Can you work these out from the model? Positions are in its coordinate system, mm. A direction names the side the tool comes from. Give positions to 0.01 mm unless a question says otherwise; leave off trailing zeros. Loops run counter-clockwise (first coordinate to the right, second up) from the corner with the lowest first, then second, coordinate; pieces in that order, holes last. Notation, with made-up numbers: M 72,79 L 123,79 A18 ccw 123,104 Z; hole C 75,7.5 d6. An arc over 180 degrees is marked long. One line per item, written item: value. Start each with the question number.
from build123d import *

# Parameters (mm, degrees)
F4_DEPTH = 2.794
F5_DEPTH = 25.4
F6_R     = 1.524
F7_DEPTH = 25.4
F9_DEPTH = 5.6388


with BuildPart() as f1:
    # F0 (on Front) → F1 (revolve)
    with BuildSketch(Plane.XZ):
        with BuildLine():
            Line((-42.70291, -13.129885), (-44.45, 0))
            Line((-44.45, 0), (-50.3936, 0))
            Line((-50.3936, 0), (-50.8, 0))
            Line((-50.8, 0), (-50.8, -0.4064))
            Line((-50.8, -0.4064), (-50.8, -5.238044))
            ThreePointArc((-50.8, -5.238044), (-50.680968, -5.525413), (-50.3936, -5.644444))
            Line((-50.3936, -5.644444), (-47.563638, -5.644444))
            ThreePointArc((-47.563638, -5.644444), (-47.006862, -5.875069), (-46.776238, -6.431844))
            Line((-46.776238, -6.431844), (-46.776238, -11.994444))
            Line((-46.776238, -11.994444), (-45.188738, -11.994444))
            Line((-45.188738, -11.994444), (-45.188738, -16.756944))
            Line((-45.188738, -16.756944), (-46.29761, -16.756944))
            ThreePointArc((-46.29761, -16.756944), (-46.558236, -16.898475), (-46.581447, -17.194142))
            Line((-46.581447, -17.194142), (-45.188738, -20.32))
            Line((-45.188738, -20.32), (-42.70291, -20.32))
            Line((-42.70291, -20.32), (-42.70291, -15.669885))
            Line((-42.70291, -15.669885), (0, -15.669885))
            Line((0, -15.669885), (0, -13.129885))
            Line((0, -13.129885), (-42.70291, -13.129885))
        make_face()
    revolve(axis=Axis((0, 0, -10.16), (0, 0, 1)))

    # F3 (on offset) → F4 (cut)
    with BuildSketch(Plane.XY.offset(-13.129885)):
        with BuildLine():
            Line((9.017678, -37.635088), (0, -37.596034))
            Line((0, -37.596034), (-9.717249, -37.55395))
            ThreePointArc((-9.717249, -37.55395), (-11.76304, -38.289364), (-12.85615, -40.168513))
            ThreePointArc((-12.85615, -40.168513), (-12.767446, -40.917369), (-12.276714, -41.489938))
            ThreePointArc((-12.276714, -41.489938), (0.021671, -44.985599), (12.224982, -41.171267))
            ThreePointArc((12.224982, -41.171267), (12.731825, -40.501367), (12.721155, -39.661401))
            ThreePointArc((12.721155, -39.661401), (11.852038, -38.366333), (10.471091, -37.641383))
            Line((10.471091, -37.641383), (9.017678, -37.635088))
        make_face()
    extrude(amount=-F4_DEPTH, mode=Mode.SUBTRACT)

    # F3 (on offset) → F5 (cut)
    with BuildSketch(Plane.XY.offset(-13.129885)):
        with BuildLine():
            ThreePointArc((1.524, 34.925), (-1.077631, 36.002631), (0, 33.401))
            ThreePointArc((0, 33.401), (1.077631, 33.847369), (1.524, 34.925))
        make_face()
        with BuildLine():
            Line((9.017678, -37.635088), (0, -37.596034))
            Line((0, -37.596034), (-9.717249, -37.55395))
            ThreePointArc((-9.717249, -37.55395), (-11.76304, -38.289364), (-12.85615, -40.168513))
            ThreePointArc((-12.85615, -40.168513), (-12.767446, -40.917369), (-12.276714, -41.489938))
            ThreePointArc((-12.276714, -41.489938), (0.021671, -44.985599), (12.224982, -41.171267))
            ThreePointArc((12.224982, -41.171267), (12.731825, -40.501367), (12.721155, -39.661401))
            ThreePointArc((12.721155, -39.661401), (11.852038, -38.366333), (10.471091, -37.641383))
            Line((10.471091, -37.641383), (9.017678, -37.635088))
        make_face()
        with BuildLine():
            ThreePointArc((10.471091, -37.641383), (9.74475, -37.55395), (9.017678, -37.635088))
            Line((9.017678, -37.635088), (10.471091, -37.641383))
        make_face()
    extrude(amount=F5_DEPTH, mode=Mode.SUBTRACT)

    # F6 (on offset) → F7 (cut)
    with BuildSketch(Plane.XY.offset(-13.129885)):
        with Locations((0, 34.925)):
            Circle(F6_R)
    extrude(amount=-F7_DEPTH, mode=Mode.SUBTRACT)

    # F8 (on Top) → F9 (join)
    with BuildSketch(Plane.XY):
        with BuildLine():
            ThreePointArc((-8.199207, 50.090913), (-4.113462, 50.596688), (0, 50.76566))
            Line((0, 50.76566), (0, 54.563351))
            Line((0, 54.563351), (-5.152237, 54.563351))
            ThreePointArc((-5.152237, 54.563351), (-5.816961, 54.375498), (-6.285039, 53.867511))
            Line((-6.285039, 53.867511), (-8.003992, 50.476065))
            Line((-8.003992, 50.476065), (-8.199207, 50.090913))
        make_face()
        with BuildLine():
            Line((0, 54.563351), (0, 50.76566))
            ThreePointArc((0, 50.76566), (4.113462, 50.596688), (8.199207, 50.090913))
            Line((8.199207, 50.090913), (8.003992, 50.476065))
            Line((8.003992, 50.476065), (6.285039, 53.867511))
            ThreePointArc((6.285039, 53.867511), (5.816961, 54.375498), (5.152237, 54.563351))
            Line((5.152237, 54.563351), (0, 54.563351))
        make_face()
        with BuildLine():
            Line((8.003992, 50.476065), (8.199207, 50.090913))
            Line((8.199207, 50.090913), (8.625197, 50.020322))
            ThreePointArc((8.625197, 50.020322), (8.260189, 50.174036), (8.003992, 50.476065))
        make_face()
        with BuildLine():
            Line((-8.625197, 50.020322), (-8.199207, 50.090913))
            Line((-8.199207, 50.090913), (-8.003992, 50.476065))
            ThreePointArc((-8.003992, 50.476065), (-8.260189, 50.174036), (-8.625197, 50.020322))
        make_face()
    extrude(amount=-F9_DEPTH)


solid = f1.part
Q1. If we section it at B-B, the plane z = -3: Write out the boundary of the cut face in (x, y).
Q2. For P1, Ø3, axis at x = -22, y = -4.5, coming from the +Z side; P2, Ø3, axis at y = -16, z = -12.5, coming from the +X side; P3, Ø1.5, axis at x = -3, z = -13.5, coming from the -Y side, each with a flat end and sliding along its axis, tell me the tip position at first contact or that it passes through.
Q3. If we mould it in two halves opening along Z, with no side actions, what happens to faces 1 (the face through (2.3, 42.75, -12.31)), 2 (the face through (10.1, 44.4, -16.757)), 3 (the face through (-7.13, 52.2, -2.78))? For each: released by +Z, released by -Z, zero draft, split by the parting line, or undercut.
Q4. I need wall thicknesses on line 1 along Y through (x, z) = (0, -14.15); line 2 along Y through (x, z) = (0, -17.8); line 3 along Y through (x, z) = (0, -17). Which ranges of each line are inside material? Lowest first, please.
Q5. Which directions (+Z, -Z, +X, -X, +Y, -Y) give clear straight access to the entire face, cutting with the end or side of a thin tool? Please do faces 4 (the face through (0, -43, -15.924)), 5 (the face through (24.5, -38.3, -11.994)), 6 (the face through (0, 52, -5.639)), 7 (the face through (9.257, 41.687, -17.962)).
Response:
1. outline: M -8.37,50.11 A50.8 ccw long 8.37,50.11 A0.85 cw 8,50.48 L 6.29,53.87 A1.27 ccw 5.15,54.56 L -5.15,54.56 A1.27 ccw -6.29,53.87 L -8,50.48 A0.85 cw Z; hole M -9.41,-43.03 A22.36 ccw 8.38,-43.25 A44.05 ccw long Z
2. P1: z = -13.13
2. P2: x = 44.44
2. P3: y = -45.13
3. face 1: released by +Z
3. face 2: undercut
3. face 3: zero draft
4. line 1: -45.19 to -44.99, -37.6 to 33.4, 36.45 to 45.19
4. line 2: -46.31 to -42.7, 42.7 to 46.31
4. line 3: -46.6 to -42.7, 42.7 to 46.6
5. face 4: +Z
5. face 5: none
5. face 6: -Z, +X, -X, +Y
5. face 7: -Z
